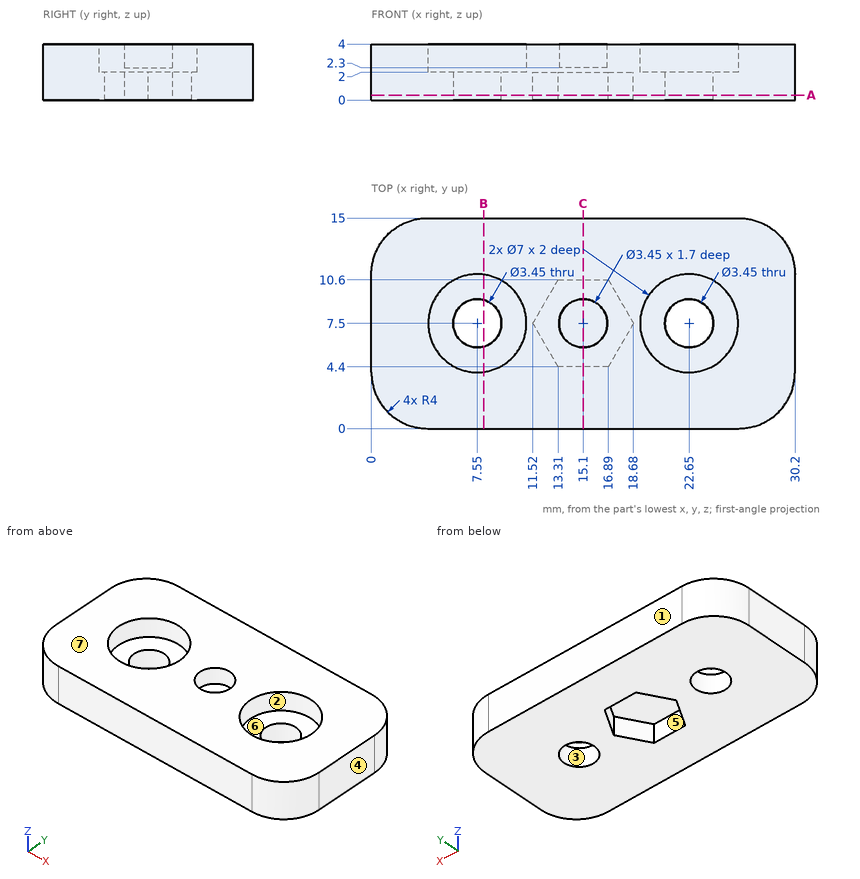
Can you work these out from the drawing? Everything is in mm from the part's minimum corner. A direction names the side the tool comes from. Give positions to 0.01 mm unless a question says otherwise; leave off trailing zeros. Order: outer loops, then holes, each group sorted by start corner. A loop starts at its lowest first (then second) coordinate and runs counter-clockwise, first axis right, second up.
1. We'd pull the mould along Y, two halves only. Please class the marked faces 1, 2, 3 and 4: pulls with the +Y half, pulls with the -Y half, needs draft (parallel to the pull), parting line crosses it, or undercut.
2. Suppose I cut it at A-A (z = 0.35). Give the number of separate pieces and of enclosed holes in the cut face, plus the area to 3 significant figures.
3. For the marked faces 5, 6 and 7, which set-ups out of +Z, -Z, +X, -X, +Y, -Y let a thin tool reach every point of the face, with its end or its side?
4. Suppose I cut it at C-C (x = 15.1). List the corners of the cut face in (y, z) for me (1 decimal).
5. Suppose I cut it at B-B (x = 8). List the corners of the cut face in (y, z) for me (1 decimal).
6. I need wall thicknesses on L1, parallel to Y at x = 7.55, z = 0.9 (1 decimal); L2, parallel to Y at x = 22.65, z = 3.5; L3, parallel to Z at x = 21, y = 6.5. Which ranges of each line are inside material? Lowest first, please.
7. Will these pins go through, and if not, where does the flat tip stop? P1, Ø2, axis at x = 22.65, y = 7.5, coming from the +Z side; P2, Ø3, axis at x = 15.1, y = 7.5, coming from the -Z side.
Solved:
1. face 1: pulls with the +Y half
1. face 2: undercut
1. face 3: undercut
1. face 4: needs draft
2. separate pieces: 1
2. enclosed holes: 3
2. area: 387 mm2
3. face 5: -Z
3. face 6: +Z
3. face 7: +Z, +X, -X, +Y, -Y
4. outline: (0, 0) - (4.4, 0) - (4.4, 2) - (10.6, 2) - (10.6, 0) - (15, 0) - (15, 4) - (9.2, 4) - (9.2, 2.3) - (5.8, 2.3) - (5.8, 4) - (0, 4) - close
5. outline: (0, 0) - (5.8, 0) - (5.8, 2) - (4, 2) - (4, 4) - (0, 4) - close; (9.2, 0) - (15, 0) - (15, 4) - (11, 4) - (11, 2) - (9.2, 2) - close
6. L1: y = 0 to 5.8, 9.2 to 15
6. L2: y = 0 to 4, 11 to 15
6. L3: z = 0 to 2
7. P1: passes through
7. P2: stops at z = 2
